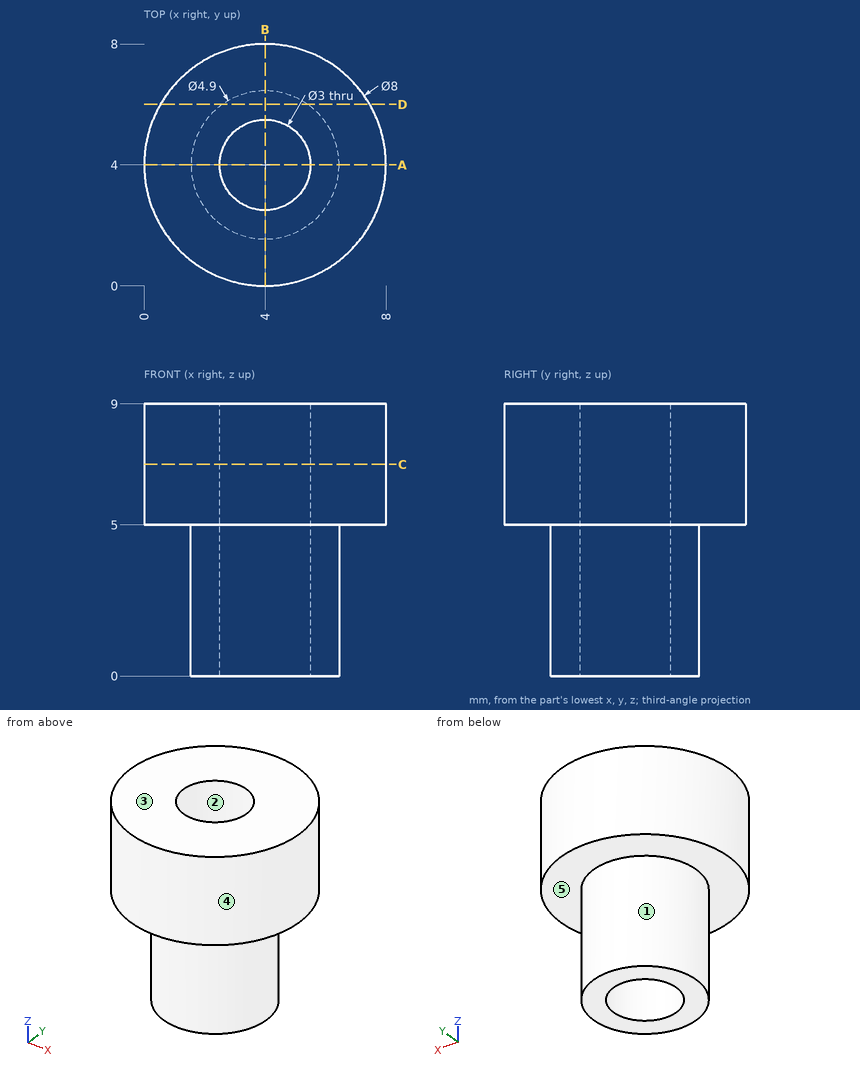
For this review, use the dimensioned drawing (mm, ordinates from the lowest corner) and the shaded views. A direction names the side the tool comes from. Round coordinates to 2 decimals unless told otherwise and drop trailing zeros. Write each loop counter-clockwise with the first axis right and the second up, starting at its lowest first coordinate (ties: lowest second). Pieces come first, ordered by that corner, then holes. Notation, with made-up numbers: (-16.5, 6) -> (2.5, 6) arc R32 cw to (2.5, 41) -> close; hole circle Ø5 at (85.5, 82.25). An arc over 180 degrees is marked (long way). Use CSV: the item, a comma, the result in double quotes.
Q1. Mouldability with a two-part tool opening along X and no side actions: class the marked faces 1, 2 and 3 as released by +X, released by -X, zero draft, split by the parting line, or undercut.
Checks:
face 1,"split by the parting line"
face 2,"undercut"
face 3,"zero draft"
Q2. Consider section D-D (y = 6). Give the boundary of the cut face in (x, z), then the cut area to 3 significant figures.
Checks:
outline,"(0.54, 5) -> (2.58, 5) -> (2.58, 0) -> (5.42, 0) -> (5.42, 5) -> (7.46, 5) -> (7.46, 9) -> (0.54, 9) -> close"
area,"41.9 mm²"
Q3. Consider section C-C (z = 7). Give the boundary of the cut face in (x, y).
Checks:
outline,"circle Ø8 at (4, 4); hole circle Ø3 at (4, 4)"
Q4. Consider section A-A (y = 4). Give the boundary of the cut face in (x, z).
Checks:
outline,"(0, 5) -> (1.55, 5) -> (1.55, 0) -> (2.5, 0) -> (2.5, 9) -> (0, 9) -> close; (5.5, 0) -> (6.45, 0) -> (6.45, 5) -> (8, 5) -> (8, 9) -> (5.5, 9) -> close"
Q5. For the marked faces 4 and 5, list the 3-axis set-ups (+Z, -Z, +X, -X, +Y, -Y) from which the entire face can be reached by the end or side of a thin tool; tool diameter is ignored.
Checks:
face 4,"+Z, -Z"
face 5,"-Z"
Q6. For pin 1 Ø4 at (x, y) = (6.5, 2.5) entering from -Z; pin 2 Ø4 at (x, z) = (4.5, 1.5) entering from -Y; pin 3 Ø4 at (x, z) = (1.5, 5.5) entering from -Y; pin 4 Ø1 at (y, z) = (2, 1.5) entering from +X, all flat-tipped, find the tip position at first contact; note any pin that passes through.
Checks:
pin 1,"z = 0"
pin 2,"y = 1.55"
pin 3,"y = 0.03"
pin 4,"x = 5.94"
Q7. To check wall thickness, follow probe 1 along Y at (x, z) = (4, 4.75); probe 2 along Y at (x, z) = (4, 6.75); probe 3 along Z at (x, y) = (2.25, 2.25). State the ranges of each line that lie inside material, in increasing order. Write a range as [from, to].
Checks:
probe 1,"[1.55, 2.5], [5.5, 6.45]"
probe 2,"[0, 2.5], [5.5, 8]"
probe 3,"[5, 9]"
